```python
from build123d import *

# Parameters (mm, degrees)
SKETCH3_R           = 12.7
BOSS_EXTRUDE1_DEPTH = 304.8
CHAMFER1_SIZE       = 2.54
CUT_EXTRUDE1_START  = -114.1
SKETCH4_R           = 12.7
CUT_EXTRUDE1_DEPTH  = 496.5
CUT_EXTRUDE2_START  = -5.08
SKETCH5_R           = 12.7
SKETCH5_R_2         = 11.938
CUT_EXTRUDE2_DEPTH  = 1.1684


with BuildPart() as part:
    # Sketch3 → Boss-Extrude1 (new body, symmetric)
    with BuildSketch(Plane.XY):
        Circle(SKETCH3_R)
    extrude(amount=BOSS_EXTRUDE1_DEPTH, both=True)

    # Chamfer1
    chamfer1_edges = [part.edges().sort_by_distance(p)[0] for p in [
        (-12.7, 0, -304.8),
        (-12.7, 0, 304.8),
    ]]
    chamfer(chamfer1_edges, length=CHAMFER1_SIZE)

    # Sketch4 → Cut-Extrude1 (cut, through all)
    with BuildSketch(Plane.XY.offset(304.8).offset(CUT_EXTRUDE1_START)):
        Circle(SKETCH4_R)
    extrude(amount=-CUT_EXTRUDE1_DEPTH, mode=Mode.SUBTRACT)

    # Sketch5 → Cut-Extrude2 (cut)
    with BuildSketch(Plane.XY.offset(304.8).offset(CUT_EXTRUDE2_START)):
        Circle(SKETCH5_R)
        Circle(SKETCH5_R_2, mode=Mode.SUBTRACT)
    cut_extrude2 = extrude(amount=-CUT_EXTRUDE2_DEPTH, mode=Mode.SUBTRACT)

    # Mirror3: Cut-Extrude2 across plane
    add(cut_extrude2.mirror(Plane.XY.offset(247.75)), mode=Mode.SUBTRACT)


solid = part.part
```
Geometry: final body of the model. Coordinates: model frame, mm. A direction names the side the tool comes from. Give positions to 0.01 mm unless a question says otherwise; leave off trailing zeros. Write each loop counter-clockwise with the first axis right and the second up, starting at its lowest first coordinate (ties: lowest second). Pieces come first, ordered by that corner, then holes.
1. Line query: probe 1 along X at (y, z) = (-7.5, 266); probe 2 along Y at (x, z) = (11, 271); probe 3 along Y at (x, z) = (6, 262). Output: solid intervals per line, ascending.
2. Pin query (flat end, axial travel): P1, Ø6, axis at y = 9, z = 219, coming from the +X side; P2, Ø1, axis at y = 6.5, z = 265.5, coming from the -X side; P3, Ø2, axis at x = -4.5, z = 262.5, coming from the -Y side. Return the tip coordinate at first contact, or that it passes through.
3. Section query A-A, the plane z = 286.5. Return loops of the section in (x, y), then the cut area to 3 significant figures.
4. Reachability of faces 1 (the flat face through (0, 0, 190.7)), 2 (the flat face through (11.2, -4.6, 299.72)) from +Z, -Z, +X, -X, +Y, -Y: full face, straight path, thin tool, end or side. Return the list, or none.
5. Draft query along Z for faces 3 (the flat face through (11.2, -4.6, 195.78)), 4 (the cylindrical face through (-2.75, -12.4, 248.46)), 5 (the conical face through (-8.16, -6.257, 304.677)). Return one class per face: released by +Z, released by -Z, zero draft, split by the parting line, or undercut.
Computed:
1. probe 1: x = -10.25 to 10.25
1. probe 2: y = -6.35 to 6.35
1. probe 3: y = -11.19 to 11.19
2. P1: stops at x = 11.19
2. P2: stops at x = -11.19
2. P3: stops at y = -12.21
3. outline: circle Ø25.4 at (0, 0)
3. area: 507 mm2
4. face 1: -Z, +X, -X, +Y, -Y
4. face 2: none
5. face 3: undercut
5. face 4: zero draft
5. face 5: released by +Z
